from build123d import *

# Parameters (mm, degrees)
F0_R      = 34.7636302152
F1_DEPTH  = 63.5
F1_TAPER  = -40
F2_T      = -6.35
F3_R      = 3.17499
F1_FACE_R = 34.7636302152
F4_DEPTH  = 63.5
F4_TAPER  = -45
F5_T      = -6.35


# Not quite as in the source:
# - a fillet or chamfer is up to 0.001 mm smaller than in the source, because OpenCascade refuses the exact size


with BuildPart() as f1:
    # F0 (on Top) → F1 (new body)
    with BuildSketch(Plane.XY):
        Circle(F0_R)
    extrude(amount=F1_DEPTH, taper=F1_TAPER)

    # F2
    f2_openings = [f1.faces().sort_by_distance(p)[0] for p in [
        (0, 0, 63.5),
    ]]
    offset(amount=F2_T, openings=f2_openings, kind=Kind.INTERSECTION)

    # F3 (radius 3.175 in the source; OpenCascade refuses exactly that, so slightly less here)
    f3_edges = [f1.edges().sort_by_distance(p)[0] for p in [
        (-88.046457, 0, 63.5),
        (-79.757121, 0, 63.5),
    ]]
    fillet(f3_edges, radius=F3_R)

    # F1_face (on face) → F4 (join)
    with BuildSketch(Plane(origin=(0, 0, 0), x_dir=(1, 0, 0), z_dir=(0, 0, -1))):
        Circle(F1_FACE_R)
    extrude(amount=F4_DEPTH, taper=F4_TAPER)

    # F5
    f5_openings = [f1.faces().sort_by_distance(p)[0] for p in [
        (0, 0, -63.5),
    ]]
    offset(amount=F5_T, openings=f5_openings, kind=Kind.INTERSECTION)


solid = f1.part
Model file for the job. Use its own axes, mm. Give positions to 0.01 mm unless a question says otherwise; leave off trailing zeros. Write each loop counter-clockwise with the first axis right and the second up, starting at its lowest first coordinate (ties: lowest second). Pieces come first, ordered by that corner, then holes. Notation, with made-up numbers: (87, 69) -> (128, 69) arc R30 ccw to (128, 103) -> close; hole circle Ø7 at (68, 5.25). An arc over 180 degrees is marked (long way). Write item = value, one per line.
(1) Slice it at C-C, the plane z = 45. Give the cut face in (x, y), then the cut area to 3 significant figures.
Determined:
outline = circle Ø145.05 at (0, 0); hole circle Ø128.47 at (0, 0)
area = 3,560 mm2
(2) Flat gauge pins, fed straight in: P1, Ø12, axis at x = -71.5, y = 63, coming from the +Z side; P2, Ø10, axis at x = -63, y = -32.5, coming from the -Z side; P3, Ø1, axis at x = 62, y = 70.5, coming from the +Z side; P4, Ø4, axis at x = 62.5, z = -24, coming from the -Y side. Where does each tip first touch, or does it go through?
Determined:
P1 = -54.53
P2 = -50.11
P3 = -58.62
P4 = through
(3) Mould opens along Z. For faces 1 (the face through (16.186, -25.387, -4.324)), 2 (the face through (-30.74, 23.57, -3.97)), 3 (the face through (-4.924, 37.501, 3.646)), 4 (the face through (0, 0, 6.35)) say: released by +Z, released by -Z, zero draft, split by the parting line, or undercut.
Determined:
face_1 = released by -Z
face_2 = undercut
face_3 = undercut
face_4 = released by +Z
(4) Slice it at A-A, the plane z = 24. Give the cut face in (x, y).
Determined:
outline = circle Ø109.8 at (0, 0); hole circle Ø93.23 at (0, 0)
(5) Probe line 1 along Z through (x, y) = (53, 26); line 2 along Y through (x, z) = (47, 35); line 3 along Z through (x, y) = (48, 50.5). List the from-to ranges inside material, lowest first.
Determined:
line_1 = -33.25 to -24.27, 28.92 to 38.8
line_2 = -43.63 to -30.16, 30.16 to 43.63
line_3 = -43.89 to -34.91, 41.6 to 51.48
